```python
from build123d import *

# Parameters (mm, degrees)
F0_R     = 3.95
F1_DEPTH = 22
F2_R     = 5.5
F3_DEPTH = 2.5
F4_R     = 7.435927
F4_R_2   = 3.75
F5_DEPTH = 0.7


with BuildPart() as f1:
    # F0 (on Top) → F1 (new body)
    with BuildSketch(Plane.XY):
        Circle(F0_R)
    extrude(amount=F1_DEPTH)

    # F2 (on Top) → F3 (join)
    with BuildSketch(Plane.XY):
        Circle(F2_R)
    extrude(amount=F3_DEPTH)


with BuildPart() as f5:
    # F4 (on Top) → F5 (new body)
    with BuildSketch(Plane.XY):
        Circle(F4_R)
        Circle(F4_R_2, mode=Mode.SUBTRACT)
    extrude(amount=F5_DEPTH)


with BuildPart() as f5_1:
    # F6: moved
    add(f5.part.moved(Location((0, 0, 20.1))))


with BuildPart() as f1_1:
    add(f1.part)

    # F7: cut F5
    add(f5_1.part, mode=Mode.SUBTRACT)


solid = f1_1.part
```
Build history of the part. All positions in model axes, mm. A direction names the side the tool comes from. Give positions to 0.01 mm unless a question says otherwise; leave off trailing zeros. Loops run counter-clockwise (first coordinate to the right, second up) from the corner with the lowest first, then second, coordinate; pieces in that order, holes last.
1) Drop flat-ended pins along their axis: P1, Ø2, axis at x = 4, z = 8.5, coming from the +Y side; P2, Ø3, axis at x = 2, z = 5.5, coming from the +Y side; P3, Ø1, axis at x = 2.5, y = -4, coming from the +Z side. Give the stop position or say it passes through.
Values follow:
P1: stops at y = 2.57
P2: stops at y = 3.92
P3: stops at z = 2.5
2) Band-saw the part on D-D on z = 13. List the corners of the cut face in (x, y), then the cut area to 3 significant figures.
Values follow:
outline: circle Ø7.9 at (0, 0)
area: 49.0 mm2
3) Probe line 1 along Z through (x, y) = (2.5, -4); line 2 along X through (y, z) = (-1, 4.25); line 3 along Y through (x, z) = (-2, 1.5). List the from-to ranges inside material, lowest first.
Values follow:
line 1: z = 0 to 2.5
line 2: x = -3.82 to 3.82
line 3: y = -5.12 to 5.12
4) 3-axis set-ups, long thin cutter, end or side, ignore diameter. For faces 1 (the face through (-3.135, -2.404, 21.392)), 2 (the face through (-3.746, 0.165, 20.445)), 3 (the face through (-1.19, -5.37, 1.23)): which of +Z, -Z, +X, -X, +Y, -Y reach the whole face in a straight line?
Values follow:
face 1: +Z
face 2: none
face 3: +Z, -Z
5) Band-saw the part on A-A on x = -2.5. List the corners of the cut face in (y, z), then the cut area to 3 significant figures.
Values follow:
outline: (-4.9, 0) - (4.9, 0) - (4.9, 2.5) - (3.06, 2.5) - (3.06, 20.1) - (2.8, 20.1) - (2.8, 20.8) - (3.06, 20.8) - (3.06, 22) - (-3.06, 22) - (-3.06, 20.8) - (-2.8, 20.8) - (-2.8, 20.1) - (-3.06, 20.1) - (-3.06, 2.5) - (-4.9, 2.5) - close
area: 143 mm2
6) Band-saw the part on B-B on y = 0. List the corners of the cut face in (x, z), then the cut area to 3 significant figures.
Values follow:
outline: (-5.5, 0) - (5.5, 0) - (5.5, 2.5) - (3.95, 2.5) - (3.95, 20.1) - (3.75, 20.1) - (3.75, 20.8) - (3.95, 20.8) - (3.95, 22) - (-3.95, 22) - (-3.95, 20.8) - (-3.75, 20.8) - (-3.75, 20.1) - (-3.95, 20.1) - (-3.95, 2.5) - (-5.5, 2.5) - close
area: 181 mm2
7) Band-saw the part on C-C on z = 1.75. List the corners of the cut face in (x, y).
Values follow:
outline: circle Ø11 at (0, 0)
